```python
from build123d import *

# Parameters (mm, degrees)
SKETCH1_W           = 80
SKETCH1_H           = 50
BOSS_EXTRUDE1_DEPTH = 10
SKETCH2_R           = 5.5
SKETCH2_R_2         = 11
CUT_EXTRUDE1_DEPTH  = 53.440442409
SKETCH3_R           = 10
CUT_EXTRUDE2_DEPTH  = 5


with BuildPart() as part:
    # Sketch1 → Boss-Extrude1 (new body)
    with BuildSketch(Plane(origin=(0, 0, 0), x_dir=(1, 0, 0), z_dir=(0, 1, 0))):
        with Locations((5, 0)):
            Rectangle(SKETCH1_W, SKETCH1_H)
    extrude(amount=BOSS_EXTRUDE1_DEPTH)

    # Sketch2 → Cut-Extrude1 (cut, through all)
    with BuildSketch(Plane(origin=(0, 10, 0), x_dir=(1, 0, 0), z_dir=(0, 1, 0))):
        with Locations(Location((-25.20025306, 15.49130346, 0), (0, 0, 270))):
            Circle(SKETCH2_R)
        with Locations(Location((35.2, 15.49130346, 0), (0, 0, 90))):
            Circle(SKETCH2_R)
        with Locations(Location((5, 11.49130346, 0), (0, 0, 270))):
            Circle(SKETCH2_R_2)
    extrude(amount=-CUT_EXTRUDE1_DEPTH, mode=Mode.SUBTRACT)

    # Sketch3 → Cut-Extrude2 (cut)
    with BuildSketch(Plane.XZ):
        with Locations(Location((5, 13, 0), (0, 0, 270))):
            Circle(SKETCH3_R)
    extrude(amount=-CUT_EXTRUDE2_DEPTH, mode=Mode.SUBTRACT)


solid = part.part
```
Work out the finished part from the listing and answer in its coordinate system (mm). A direction names the side the tool comes from. Give positions to 0.01 mm unless a question says otherwise; leave off trailing zeros. Loops run counter-clockwise (first coordinate to the right, second up) from the corner with the lowest first, then second, coordinate; pieces in that order, holes last. Notation, with made-up numbers: M -7.75,-6.5 L 34.25,-6.5 A3 cw 34.25,-1.5 Z; hole C 39.5,66.25 d4. An arc over 180 degrees is marked long. One line per item, written item: value. Start each with the question number.
1. Find section C-C (y = 4). Give the vertices of the cut face in (x, z).
2. Each of these flat-tipped pins is pushed along its axis until it touches: P1, Ø1, axis at x = 36.5, z = -6.5, coming from the -Y side; P2, Ø1, axis at x = 14, z = -10, coming from the -Y side. Where does it stop, or does it pass through?
3. Determine the mould class of faces 1 (the face through (45, 5, 0)), 2 (the face through (4, 5, 25)), 3 (the face through (-20.563, 5.07, -12.535)), 4 (the face through (29.747, 5.07, -14.775)) for opening direction X: released by +X, released by -X, zero draft, split by the parting line, or undercut.
4. Find section A-A (x = 35.2). Give the vertices of the cut face in (y, z).
5. Find section B-B (z = 13). Give the vertices of the cut face in (x, y).
6. Find section D-D (z = -7.5). Give the vertices of the cut face in (x, y).
7. Find the intervals of material crossed by probe 1 along Z at (x, y) = (4.5, 8.25); probe 2 along X at (y, z) = (1.95, 13); probe 3 along X at (y, z) = (1.75, -14.5), in increasing order.
8. Which of the six approach directions +Z, -Z, +X, -X, +Y, -Y give full straight-line access (tool end or side, diameter ignored) to faces 5 (the face through (0.79, 5.07, -1.33)), 6 (the face through (5, 5, 13))?
Reported:
1. outline: M -35,-25 L 45,-25 L 45,25 L -35,25 Z; hole C -25.2,-15.49 d11; hole C 5,-11.49 d22; hole C 5,13 d20; hole C 35.2,-15.49 d11
2. P1: stops at y = 0
2. P2: passes through
3. face 1: released by +X
3. face 2: zero draft
3. face 3: undercut
3. face 4: undercut
4. outline: M 0,-25 L 10,-25 L 10,-20.99 L 0,-20.99 Z; M 0,-9.99 L 10,-9.99 L 10,25 L 0,25 Z
5. outline: M -35,0 L -5,0 L -5,5 L 15,5 L 15,0 L 45,0 L 45,10 L -35,10 Z
6. outline: M -35,0 L -5.25,0 L -5.25,10 L -35,10 Z; M 15.25,0 L 45,0 L 45,10 L 15.25,10 Z
7. probe 1: z = -25 to -22.48, -0.5 to 25
7. probe 2: x = -35 to -5, 15 to 45
7. probe 3: x = -35 to -30.61, -19.79 to -5.58, 15.58 to 29.79, 40.61 to 45
8. face 5: +Y, -Y
8. face 6: -Y
